```python
from build123d import *

# Parameters (mm, degrees)
SKETCH1_W                                           = 16.25
SKETCH1_H                                           = 3.65
BOSS_EXTRUDE1_DEPTH                                 = 7.44
CBORE_FOR_00_BINDING_HEAD_MACHINE_SCREW_D           = 1.5113
CBORE_FOR_00_BINDING_HEAD_MACHINE_SCREW_DEPTH       = 5
CBORE_FOR_00_BINDING_HEAD_MACHINE_SCREW_CBORE_D     = 3.175
CBORE_FOR_00_BINDING_HEAD_MACHINE_SCREW_CBORE_DEPTH = 0.7112
CBORE_FOR_00_BINDING_HEAD_MACHINE_SCREW_TIP         = 0.454040327


with BuildPart() as part:
    # Sketch1 → Boss-Extrude1 (new body)
    with BuildSketch(Plane.XY):
        with Locations((0, 1.825)):
            Rectangle(SKETCH1_W, SKETCH1_H)
    extrude(amount=BOSS_EXTRUDE1_DEPTH)

    # CBORE for #00 Binding Head Machine Screw1
    with Locations(Plane.XY.offset(7.44)):
        with Locations((-4.873259483, 1.85), (5.126740517, 1.85)):
            CounterBoreHole(CBORE_FOR_00_BINDING_HEAD_MACHINE_SCREW_D / 2, CBORE_FOR_00_BINDING_HEAD_MACHINE_SCREW_CBORE_D / 2, CBORE_FOR_00_BINDING_HEAD_MACHINE_SCREW_CBORE_DEPTH, depth=CBORE_FOR_00_BINDING_HEAD_MACHINE_SCREW_DEPTH)
            with Locations((0, 0, -(CBORE_FOR_00_BINDING_HEAD_MACHINE_SCREW_DEPTH + CBORE_FOR_00_BINDING_HEAD_MACHINE_SCREW_TIP / 2))):  # 118° drill point
                Cone(0, CBORE_FOR_00_BINDING_HEAD_MACHINE_SCREW_D / 2, CBORE_FOR_00_BINDING_HEAD_MACHINE_SCREW_TIP, mode=Mode.SUBTRACT)


solid = part.part
```
Source: CAD feature listing. Evaluate the final solid. Frame: model axes, mm. A direction names the side the tool comes from. Give positions to 0.01 mm unless a question says otherwise; leave off trailing zeros. Loops run counter-clockwise (first coordinate to the right, second up) from the corner with the lowest first, then second, coordinate; pieces in that order, holes last. Notation, with made-up numbers: (47, 84.5) -> (82, 84.5) arc R25 ccw to (82, 108.5) -> close; hole circle Ø10 at (-20.5, 11.25). An arc over 180 degrees is marked (long way). Put each result on its own line as item: value. Start each with the question number.
1) Cut plane D-D (y = 3.1). Return loops of the section in (x, z) (3 decimals).
2) Cut plane A-A (z = 3.5). Return loops of the section in (x, y) (3 decimals).
3) Contact query for a flat-ended pin moving along its axis: P1, Ø1.7, axis at x = 5.13, y = 1.85, coming from the +Z side. Output: stop coordinate, or through.
4) Cut plane B-B (x = 3.75). Return loops of the section in (y, z).
5) Draft query along Y for faces 3 (the face through (0, 3.65, 4)), 4 (the face through (0, 2, 0)), 5 (the face through (-4.977, 1.77, 2.065)). Return one class per face: released by +Y, released by -Y, zero draft, split by the parting line, or undercut.
6) Reachability of faces 1 (the face through (0, 0, 4)), 2 (the face through (-4.316, 2.361, 4.554)) from +Z, -Z, +X, -X, +Y, -Y: full face, straight path, thin tool, end or side. Return the list, or none.
7) Material intervals for probe 1 along X at (y, z) = (1.85, 4.25) (3 decimals); probe 2 along X at (y, z) = (2.5, 2.5) (3 decimals); probe 3 along Z at (x, y) = (-3.75, 1.75), sorted ascending.
8) Cut plane C-C (y = 0.45). Return loops of the section in (x, z) (3 decimals).
Results are:
1. outline: (-8.125, 0) -> (8.125, 0) -> (8.125, 7.44) -> (6.105, 7.44) -> (6.105, 6.729) -> (4.148, 6.729) -> (4.148, 7.44) -> (-3.895, 7.44) -> (-3.895, 6.729) -> (-5.852, 6.729) -> (-5.852, 7.44) -> (-8.125, 7.44) -> close
2. outline: (-8.125, 0) -> (8.125, 0) -> (8.125, 3.65) -> (-8.125, 3.65) -> close; hole circle Ø1.511 at (-4.873, 1.85); hole circle Ø1.511 at (5.127, 1.85)
3. P1: stops at z = 6.73
4. outline: (0, 0) -> (3.65, 0) -> (3.65, 7.44) -> (2.64, 7.44) -> (2.64, 6.73) -> (1.06, 6.73) -> (1.06, 7.44) -> (0, 7.44) -> close
5. face 3: released by +Y
5. face 4: zero draft
5. face 5: undercut
6. face 1: +Z, -Z, +X, -X, -Y
6. face 2: +Z
7. probe 1: x = -8.125 to -5.629, -4.118 to 4.371, 5.882 to 8.125
7. probe 2: x = -8.125 to -5.259, -4.488 to 4.741, 5.512 to 8.125
7. probe 3: z = 0 to 6.73
8. outline: (-8.125, 0) -> (8.125, 0) -> (8.125, 7.44) -> (5.875, 7.44) -> (5.875, 6.729) -> (4.378, 6.729) -> (4.378, 7.44) -> (-4.125, 7.44) -> (-4.125, 6.729) -> (-5.622, 6.729) -> (-5.622, 7.44) -> (-8.125, 7.44) -> close
